For this review, take the finished solid that the model builds, in its own axes (mm). Face numbers are marked on the shaded views. A direction names the side the tool comes from. Round coordinates to 2 decimals unless told otherwise and drop trailing zeros. Loops run counter-clockwise (first coordinate to the right, second up) from the corner with the lowest first, then second, coordinate; pieces in that order, holes last. Notation, with made-up numbers: M 9,-28.75 L 16,-28.75 A8 cw 16,-14.75 Z; hole C -36,41 d2. An arc over 180 degrees is marked long. Write item = value, one per line. Start each with the question number.
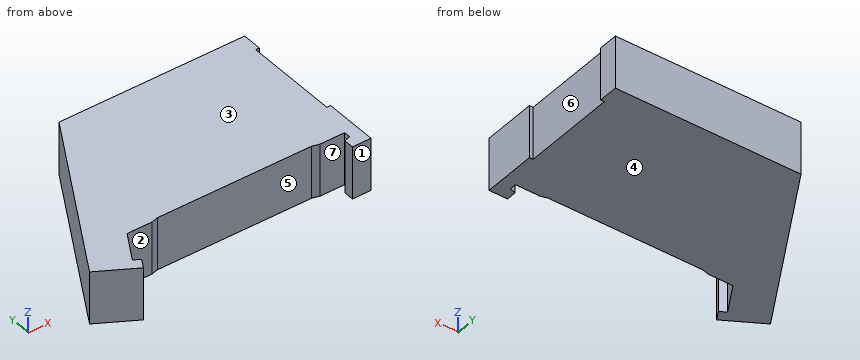
```python
from build123d import *

# Parameters (mm, degrees)
DODANIE_WYCI_GNI_CIE1_DEPTH = 8.5


with BuildPart() as part:
    # Szkic1 → Dodanie-wyciągnięcie1 (new body)
    with BuildSketch(Plane(origin=(0, 0, 0), x_dir=(-1, 0, 0), z_dir=(0, 0, -1))):
        Polygon((-8.080384758, 0.3), (16.880384758, 0.3), (18, 0), (22, 0), (24.8, -4.849742261), (23.759936491, -5.450223208), (24.659936491, -7.009068935), (30.722114317, -3.509068935), (14.839745962, 24), (-15.2, 24), (-15.2, 20.85), (-14.6, 20.85), (-14.6, 5.65), (-15.2, 5.65), (-15.2, -3), (-12.2, -3), (-12.2, -1.367949192), (-13.2, -1.1), (-13.2, 0), (-9.2, 0), align=None)
    extrude(amount=-DODANIE_WYCI_GNI_CIE1_DEPTH)


solid = part.part
```
(1) Add section D-D on y = 2.5. Write out the cut boundary in (x, z).
(2) Add section A-A on y = -2. Write out the cut boundary in (x, z), and give its area (3 significant figures).
(3) Wall thickness on L1, parallel to Y at x = 3.5, z = 6.75; L2, parallel to Y at x = 10.5, z = 0.75; L3, parallel to X at y = 12.5, z = 2.5: over which ranges is each line inside the solid? List them lowest first.
(4) Add section B-B on z = 4.5. Write out the cut boundary in (x, y), and give its area (3 significant figures).
(5) Draft analysis for pull direction Y (two halves, no side actions). For the marked faces 4, 5, 6 and 7, state which applies: +Y half, -Y half, draft (parallel to the pull), parting line (faces both ways), or undercut.
(6) For pin 1 Ø3 at (x, z) = (-20, 6) entering from -Y; pin 2 Ø4 at (y, z) = (16, 5) entering from +X; pin 3 Ø3.5 at (x, z) = (13.5, 2) entering from -Y, all flat-tipped, find the tip position at first contact; note any pin that passes through.
(7) Add section C-C on x = -12. Write out the cut boundary in (y, z).
(8) Tool access review of the marked faces 1, 2 and 3: name each direction out of +Z, -Z, +X, -X, +Y, -Y from which nothing blocks a thin tool from reaching the whole face with its end or side.
Answer sheet:
q1.outline = M -27.25,0 L 15.2,0 L 15.2,8.5 L -27.25,8.5 Z
q2.outline = M -29.85,0 L -23.15,0 L -23.15,8.5 L -29.85,8.5 Z; M 12.2,0 L 15.2,0 L 15.2,8.5 L 12.2,8.5 Z
q2.area = 82.4 mm²
q3.L1 = 0.3 to 24
q3.L2 = 0 to 24
q3.L3 = -21.48 to 14.6
q4.outline = M -30.72,-3.51 L -24.66,-7.01 L -23.76,-5.45 L -24.8,-4.85 L -22,0 L -18,0 L -16.88,0.3 L 8.08,0.3 L 9.2,0 L 13.2,0 L 13.2,-1.1 L 12.2,-1.37 L 12.2,-3 L 15.2,-3 L 15.2,5.65 L 14.6,5.65 L 14.6,20.85 L 15.2,20.85 L 15.2,24 L -14.84,24 Z
q4.area = 913 mm²
q5.face_4 = draft
q5.face_5 = -Y half
q5.face_6 = undercut
q5.face_7 = undercut
q6.pin_1 = 0
q6.pin_2 = 14.6
q6.pin_3 = -3
q7.outline = M 0.3,0 L 24,0 L 24,8.5 L 0.3,8.5 Z
q8.face_1 = +Z, -Z, +X, -Y
q8.face_2 = +Z, -Z, -Y
q8.face_3 = +Z, +X, -X, +Y, -Y
